Check sheet for the drawn part. Datum: minimum x, y, z corner. Units: mm. Give positions to 0.01 mm unless a question says otherwise; leave off trailing zeros. Write each loop counter-clockwise with the first axis right and the second up, starting at its lowest first coordinate (ties: lowest second). Pieces come first, ordered by that corner, then holes.
(1) Thickness scan on line 1 along Z through (x, y) = (3, 1.55) (1 decimal); line 2 along Z through (x, y) = (5.75, 1.3) (1 decimal); line 3 along X through (y, z) = (4.8, 7.75). Record the ranges inside material, lowest first.
(2) Cross-section at C-C (x = 6.75). Record the boundary of the cut face in (y, z).
(3) Cross-section at D-D (x = 9.5). Record the boundary of the cut face in (y, z).
(4) Mould release check, pull along Z, two halves, no side actions. Record for the marked faces 1, 2, 3 and 4: +Z half, -Z half, draft (parallel to the pull), parting line (faces both ways), or undercut.
(5) Cross-section at A-A (z = 3.5). Record the boundary of the cut face in (x, y).
(6) Depth check by flat-ended pin: P1, Ø2, axis at y = 1, z = 2.5, coming from the -X side. Enter the tip coordinate at first touch or a pass-through.
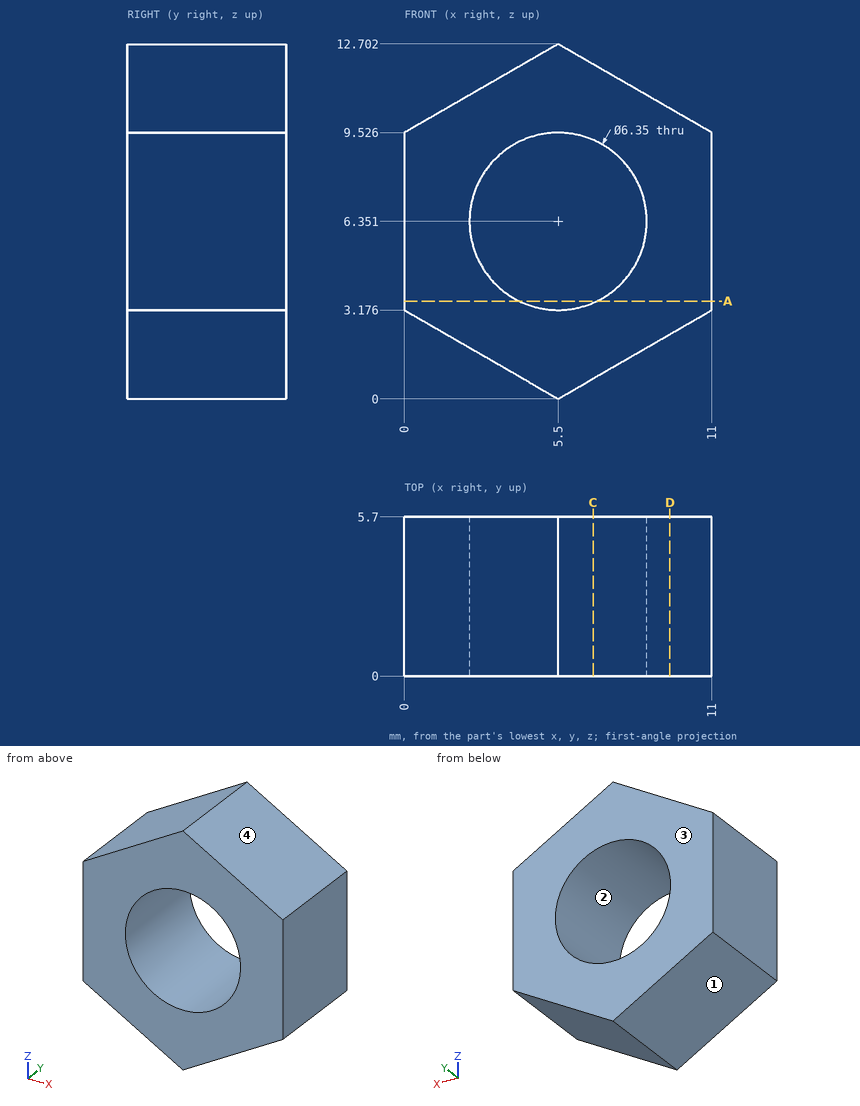
Reply:
1. line 1: z = 1.4 to 4.4, 8.3 to 11.3
1. line 2: z = 0.1 to 3.2, 9.5 to 12.6
1. line 3: x = 0 to 2.65, 8.35 to 11
2. outline: (0, 0.72) - (5.7, 0.72) - (5.7, 3.43) - (0, 3.43) - close; (0, 9.27) - (5.7, 9.27) - (5.7, 11.98) - (0, 11.98) - close
3. outline: (0, 2.31) - (5.7, 2.31) - (5.7, 10.39) - (0, 10.39) - close
4. face 1: -Z half
4. face 2: undercut
4. face 3: draft
4. face 4: +Z half
5. outline: (0, 0) - (4.1, 0) - (4.1, 5.7) - (0, 5.7) - close; (6.9, 0) - (11, 0) - (11, 5.7) - (6.9, 5.7) - close
6. P1: stops at x = 0
